Autodesk Inventor part; units mm, degrees
ref_plane "YZ Plane" through (0, 0, 0) normal (1, 0, 0) x (0, 1, 0)
ref_plane "XZ Plane" through (0, 0, 0) normal (0, 1, 0) x (-1, 0, 0)
ref_plane "XY Plane" through (0, 0, 0) normal (0, 0, 1) x (1, 0, 0)
sketch "Sketch1" plane through (0, 0, 0) normal (0, 0, 1) x (1, 0, 0)
  circle A0 centre (0, 0) radius 29.972
  circle A1 centre (0, 0) radius 25.4 construction
  circle A2 centre (12.7, 21.997) radius 2.5527 construction
  circle A3 centre (-12.7, 21.997) radius 2.5527 construction
  circle A4 centre (-25.4, 0) radius 2.5527 construction
  circle A5 centre (-12.7, -21.997) radius 2.5527 construction
  circle A6 centre (12.7, -21.997) radius 2.5527 construction
  circle A7 centre (25.4, 0) radius 2.5527 construction
  line L0 (-12.7, 21.997) -> (12.7, 21.997) construction
  arc A8 (-14.986, 25.9565) -> (-10.414, 18.0376) centre (-12.7, 21.997) ccw
  arc A9 (-10.414, -18.0376) -> (-10.414, 18.0376) centre (0, 0) ccw
  arc A10 (-10.414, -18.0376) -> (-14.986, -25.9565) centre (-12.7, -21.997) ccw
  dimension "d1" = 50.8
  dimension "d0" = 59.944
  dimension "d2" = 5.1054
  dimension "d5" = 360
extrude "Extrusion1" add sketch "Sketch1" along normal blind 25.4 contours A0 A10 A9 A8 picked at (-11.332, -24.2357)
sketch "Sketch2" plane through (0, 0, 0) normal (0, 0, -1) x (-1, 0, 0)
  circle A0 centre (0, 0) radius 29.972
  circle A1 centre (0, 0) radius 9.8425
  arc A2 (14.986, 25.9565) -> (14.986, -25.9565) centre (0, 0) ccw
  dimension "d13" = 19.685
  dimension "d14" = 59.944
extrude "Extrusion2" add sketch "Sketch2" along normal blind 3.81
sketch "Sketch3" plane through (0, 0, 25.4) normal (0, 0, 1) x (1, 0, 0)
  circle A0 centre (0, 0) radius 9.8425
  circle A1 centre (0, 0) radius 25.4
  arc A2 (-14.986, 25.9565) -> (-10.414, 18.0376) centre (-12.7, 21.997) ccw
  point P0 (-25.4, 0)
  point P1 (-12.7, -21.997)
  point P2 (12.7, -21.997)
  point P3 (25.4, 0)
  point P4 (12.7, 21.997)
  dimension "d19" = 360
hole "Hole1" at (-12.7, 21.997, 25.4) at (12.7, 21.997, 25.4) at (25.4, 0, 25.4) at (12.7, -21.997, 25.4) at (-12.7, -21.997, 25.4) direction (0, 0, -1) diameter 5.1054 end through all
properties part number "Motor_spacer_Falcon"
Here's how the part is built. I have some questions about the finished solid (model axes, mm). A direction names the side the tool comes from. Round coordinates to 2 decimals unless told otherwise and drop trailing zeros. Loops run counter-clockwise (first coordinate to the right, second up) from the corner with the lowest first, then second, coordinate; pieces in that order, holes last.
1. If we section it at D-D on y = 9: Write out the boundary of the cut face in (x, z), plus the area to 3 significant figures.
Answer list:
outline: (-28.59, -3.81) - (-3.98, -3.81) - (-3.98, 0) - (-28.59, 0) - close; (3.98, -3.81) - (28.59, -3.81) - (28.59, 25.4) - (18.78, 25.4) - (18.78, 0) - (3.98, 0) - close
area: 437 mm2
2. If we section it at B-B on z = 13: Write out the boundary of the cut face in (x, y), plus the area to 3 significant figures.
Answer list:
outline: (-14.99, -25.96) arc R29.97 ccw (long way) to (-14.99, 25.96) arc R4.57 ccw to (-10.41, 18.04) arc R20.83 cw (long way) to (-10.41, -18.04) arc R4.57 ccw to start; hole circle Ø5.11 at (-12.7, -22); hole circle Ø5.11 at (-12.7, 22); hole circle Ø5.11 at (12.7, -22); hole circle Ø5.11 at (12.7, 22); hole circle Ø5.11 at (25.4, 0)
area: 936 mm2
3. If we section it at A-A on x = 0: Write out the boundary of the cut face in (y, z).
Answer list:
outline: (-29.97, -3.81) - (-9.84, -3.81) - (-9.84, 0) - (-20.83, 0) - (-20.83, 25.4) - (-29.97, 25.4) - close; (9.84, -3.81) - (29.97, -3.81) - (29.97, 25.4) - (20.83, 25.4) - (20.83, 0) - (9.84, 0) - close
4. We'd pull the mould along Y, two halves only. Please class faces 3 (the face through (-29.97, 0.44, -1.88)), 4 (the face through (-11.722, -24.355, 10.591)), 5 (the face through (7.1, 7.1, -3.81)): +Y half, -Y half, draft (parallel to the pull), parting line (faces both ways), or undercut.
Answer list:
face 3: parting line
face 4: undercut
face 5: draft
5. If I drill on line 1 along Y through (x, z) = (12.7, 16.5); line 2 along Y through (x, z) = (0, 10); line 3 along Z through (x, y) = (11.5, -15.5), over which ranges is the centre line in solid material (lowest first)?
Answer list:
line 1: y = -27.15 to -24.55, -19.44 to -16.51, 16.51 to 19.44, 24.55 to 27.15
line 2: y = -29.97 to -20.83, 20.83 to 29.97
line 3: z = -3.81 to 0
6. If we section it at C-C on x = 12.7: Write out the boundary of the cut face in (y, z), plus the area to 3 significant figures.
Answer list:
outline: (-27.15, -3.81) - (-24.55, -3.81) - (-24.55, 25.4) - (-27.15, 25.4) - close; (-19.44, -3.81) - (19.44, -3.81) - (19.44, 25.4) - (16.51, 25.4) - (16.51, 0) - (-16.51, 0) - (-16.51, 25.4) - (-19.44, 25.4) - close; (24.55, -3.81) - (27.15, -3.81) - (27.15, 25.4) - (24.55, 25.4) - close
area: 449 mm2
7. For P1, Ø5, axis at y = -22, z = 6, coming from the +X side; P2, Ø6.5, axis at x = 25.4, y = 0, coming from the -Z side; P3, Ø8, axis at x = 17, z = 16.5, coming from the -Y side; P4, Ø22.5, axis at x = 0, y = 0, coming from the +Z side, each with a flat end and sliding along its axis, tell me the tip position at first contact or that it passes through.
Answer list:
P1: stops at x = 22.76
P2: stops at z = -3.81
P3: stops at y = -27.01
P4: stops at z = 0
8. Which directions (+Z, -Z, +X, -X, +Y, -Y) give clear straight access to the entire face, cutting with the end or side of a thin tool? Please do faces 1 (the face through (-16.608, 19.625, 12.522)), 2 (the face through (13.678, -24.355, 10.591)).
Answer list:
face 1: +Z
face 2: +Z, -Z
